```python
from build123d import *

# Parameters (mm, degrees)
F0_W     = 1400
F0_H     = 700
F0_W_2   = 50
F0_H_2   = 50
F1_DEPTH = 120
F2_R     = 10
F3_DEPTH = 1000


with BuildPart() as f1:
    # F0 (on Top) → F1 (new body)
    with BuildSketch(Plane.XY):
        with Locations((-1542.525277, -310)):
            Rectangle(F0_W, F0_H)
        with Locations((-2177.525277, -595)):
            Rectangle(F0_W_2, F0_H_2, mode=Mode.SUBTRACT)
        with Locations((-907.525277, -595)):
            Rectangle(F0_W_2, F0_H_2, mode=Mode.SUBTRACT)
        with Locations((-2177.525277, -25)):
            Rectangle(F0_W_2, F0_H_2, mode=Mode.SUBTRACT)
        Polygon((-2202.525277, -530), (-2202.525277, -90), (-2112.525277, -90), (-2112.525277, 0), (-972.525277, 0), (-972.525277, -90), (-882.525277, -90), (-882.525277, -530), (-972.525277, -530), (-972.525277, -620), (-2112.525277, -620), (-2112.525277, -530), align=None, mode=Mode.SUBTRACT)
        with Locations((-907.525277, -25)):
            Rectangle(F0_W_2, F0_H_2, mode=Mode.SUBTRACT)
    extrude(amount=F1_DEPTH)

    # F2 (on face) → F3 (cut)
    with BuildSketch(Plane.XZ.offset(660)):
        with Locations((-2177.525277, 50)):
            Circle(F2_R)
    extrude(amount=-F3_DEPTH, mode=Mode.SUBTRACT)


solid = f1.part
```
Source: CAD feature listing. Evaluate the final solid. Frame: model axes, mm. Round coordinates to 2 decimals unless told otherwise and drop trailing zeros. Loops run counter-clockwise (first coordinate to the right, second up) from the corner with the lowest first, then second, coordinate; pieces in that order, holes last. Notation, with made-up numbers: M 4.5,65 L 16.5,65 A21 cw 16.5,101 Z; hole C -33.75,-7.75 d7. An arc over 180 degrees is marked long. Put each result on its own line as item: value.
(1) Ray query, line 1 (Y direction, x = -1357, z = 11.5); line 2 (X direction, y = -274.5, z = 114). Return the intervals inside material, ascending. Write a range as [from, to].
Solutions:
line 1: [-660, -620], [0, 40]
line 2: [-2242.53, -2202.53], [-882.53, -842.53]
(2) Section A-A, the plane y = -215.5. Return loops of the section in (x, z), and give its area (3 significant figures).
Solutions:
outline: M -2242.53,0 L -2202.53,0 L -2202.53,120 L -2242.53,120 Z; M -882.53,0 L -842.53,0 L -842.53,120 L -882.53,120 Z
area: 9,600 mm²
(3) Section C-C, the plane z = 13. State how many separate pieces and enclosed holes the cut face has, and give its area (3 significant figures).
Solutions:
separate pieces: 1
enclosed holes: 5
area: 184,000 mm²
(4) Pull-direction query (Y, two-part tool) for faces 1 (the face through (-2242.525, -315, 59)), 2 (the face through (-2112.525, -46, 59)); classes: released by +Y, released by -Y, zero draft, split by the parting line, or undercut.
Solutions:
face 1: zero draft
face 2: undercut
(5) Section B-B, the plane x = -2037.5. Return loops of the section in (y, z), and give its area (3 significant figures).
Solutions:
outline: M -660,0 L -620,0 L -620,120 L -660,120 Z; M 0,0 L 40,0 L 40,120 L 0,120 Z
area: 9,600 mm²
